For this review, use the dimensioned drawing (mm, ordinates from the lowest corner) and the shaded views. Round coordinates to 2 decimals unless told otherwise and drop trailing zeros. Loops run counter-clockwise (first coordinate to the right, second up) from the corner with the lowest first, then second, coordinate; pieces in that order, holes last. Notation, with made-up numbers: M 87.25,6 L 119.25,6 A31 cw 119.25,33 Z; hole C -18.5,49.5 d5. An arc over 180 degrees is marked long. Use a Markdown table: item, result. Add a question column.
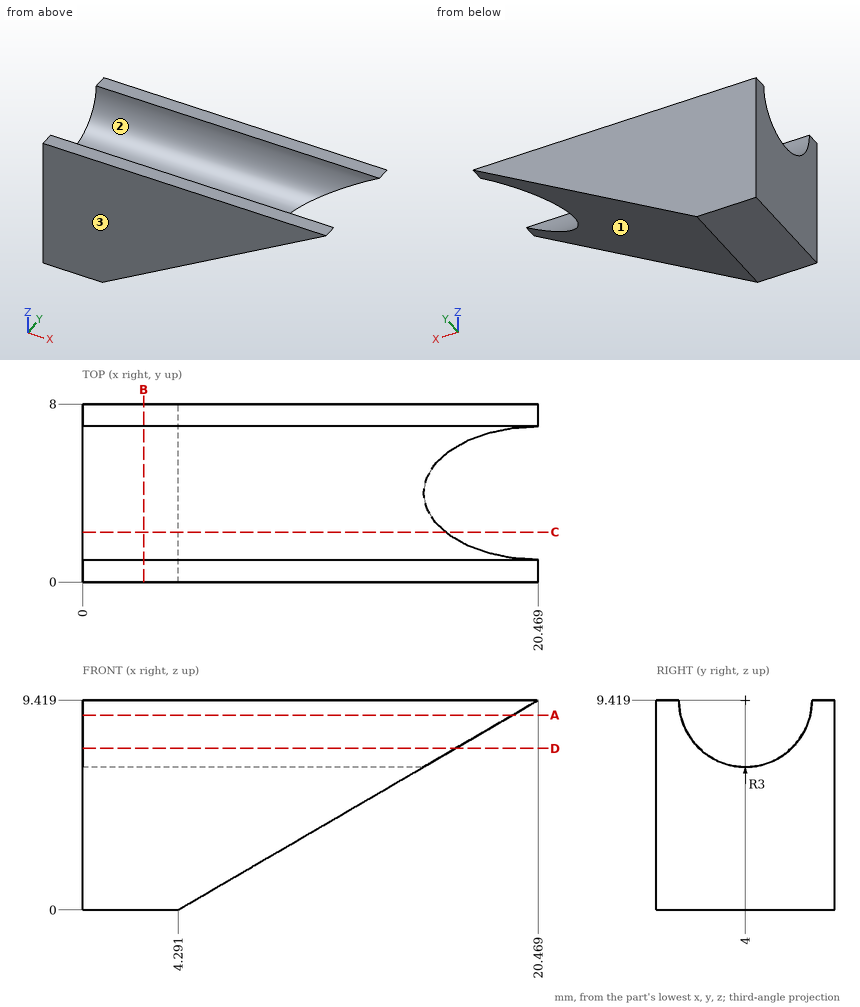
(1) Consider section C-C, the plane y = 2.25. Give the boundary of the cut face in (x, z).
(2) Draft analysis for pull direction Y (two halves, no side actions). For the marked faces 1, 2 and 3, state which applies: released by +Y, released by -Y, zero draft, split by the parting line, or undercut.
(3) Consider section B-B, the plane x = 2.75. Give the boundary of the cut face in (y, z), then the cut area to 3 significant figures.
(4) To check wall thickness, follow probe 1 along Y at (x, z) = (3.75, 7.25); probe 2 along X at (y, z) = (1.5, 2.75) (1 decimal); probe 3 along Z at (x, y) = (7.75, 2) (1 decimal). State the ranges of each line that lie inside material, in increasing order.
(5) Consider section D-D, the plane z = 7.25. Give the boundary of the cut face in (x, y).
(6) Insertion check: pin 1 Ø4 at (y, z) = (4, 3) entering from +X. The pin has a flat end and moves straight along its axis. Give the tip position at first contact, or say it passes through.
(7) Consider section A-A, the plane z = 8.75. Give the boundary of the cut face in (x, y) (1 decimal).
Found:
| question | item | result |
|---|---|---|
| 1 | outline | M 0,0 L 4.29,0 L 16.28,6.98 L 0,6.98 Z |
| 2 | face 1 | zero draft |
| 2 | face 2 | undercut |
| 2 | face 3 | released by -Y |
| 3 | outline | M 0,0 L 8,0 L 8,9.42 L 7,9.42 A3 cw 1,9.42 L 0,9.42 Z |
| 3 | area | 61.2 mm^2 |
| 4 | probe 1 | y = 0 to 1.93, 6.07 to 8 |
| 4 | probe 2 | x = 0 to 9 |
| 4 | probe 3 | z = 2 to 7.2 |
| 5 | outline | M 0,0 L 16.74,0 L 16.74,1.93 L 0,1.93 Z; M 0,6.07 L 16.74,6.07 L 16.74,8 L 0,8 Z |
| 6 | pin 1 | stops at x = 12.88 |
| 7 | outline | M 0,0 L 19.3,0 L 19.3,1.1 L 0,1.1 Z; M 0,6.9 L 19.3,6.9 L 19.3,8 L 0,8 Z |
